Geometry: final body of the model. Coordinates: model frame, mm. Face numbers are marked on the shaded views. A direction names the side the tool comes from. Coordinates: 2 decimals unless noted, no trailing zeros. Order: outer loops, then holes, each group sorted by start corner. A loop starts at its lowest first (then second) coordinate and runs counter-clockwise, first axis right, second up. Notation, with made-up numbers: (-36, -31.5) - (10, -31.5) arc R14 ccw to (10, -5.5) - close; hole circle Ø3 at (84, -4.5). An arc over 180 degrees is marked (long way). Use a Markdown table: item, result. Add a question column.
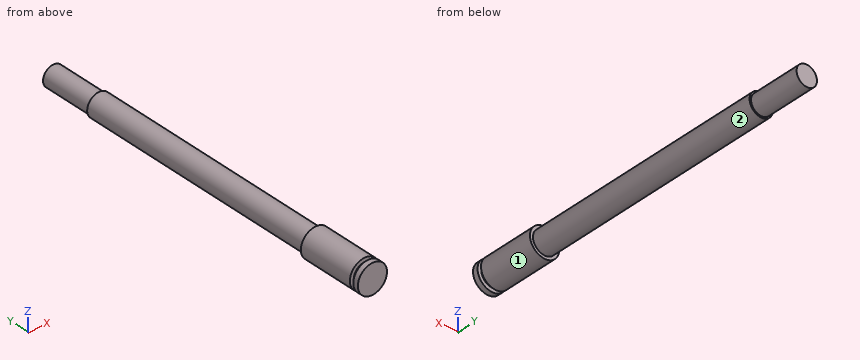
```python
from build123d import *

# Parameters (mm, degrees)
SKETCH1_R           = 5.65
BOSS_EXTRUDE1_DEPTH = 2
SKETCH2_R           = 4.15
BOSS_EXTRUDE2_DEPTH = 1.5
SKETCH3_R           = 5.65
BOSS_EXTRUDE3_DEPTH = 21.5
SKETCH4_R           = 4.5
BOSS_EXTRUDE4_DEPTH = 30
SKETCH5_R           = 4.5
BOSS_EXTRUDE5_DEPTH = 65
SKETCH6_R           = 3.95
BOSS_EXTRUDE6_DEPTH = 20


with BuildPart() as part:
    # Sketch1 → Boss-Extrude1 (new body)
    with BuildSketch(Plane(origin=(0, 0, 0), x_dir=(1, 0, 0), z_dir=(0, 1, 0))):
        with Locations(Location((0, 0, 0), (0, 0, 270))):
            Circle(SKETCH1_R)
    extrude(amount=BOSS_EXTRUDE1_DEPTH)

    # Sketch2 → Boss-Extrude2 (add)
    with BuildSketch(Plane(origin=(0, 2, 0), x_dir=(1, 0, 0), z_dir=(0, 1, 0))):
        with Locations(Location((0, 0, 0), (0, 0, 270))):
            Circle(SKETCH2_R)
    extrude(amount=BOSS_EXTRUDE2_DEPTH)

    # Sketch3 → Boss-Extrude3 (add)
    with BuildSketch(Plane(origin=(0, 3.5, 0), x_dir=(1, 0, 0), z_dir=(0, 1, 0))):
        with Locations(Location((0, 0, 0), (0, 0, 270))):
            Circle(SKETCH3_R)
    extrude(amount=BOSS_EXTRUDE3_DEPTH)

    # Sketch4 → Boss-Extrude4 (add)
    with BuildSketch(Plane(origin=(0, 25, 0), x_dir=(1, 0, 0), z_dir=(0, 1, 0))):
        with Locations(Location((0, 0, 0), (0, 0, 270))):
            Circle(SKETCH4_R)
    extrude(amount=BOSS_EXTRUDE4_DEPTH)

    # Sketch5 → Boss-Extrude5 (add)
    with BuildSketch(Plane(origin=(0, 55, 0), x_dir=(1, 0, 0), z_dir=(0, 1, 0))):
        with Locations(Location((0, 0, 0), (0, 0, 270))):
            Circle(SKETCH5_R)
    extrude(amount=BOSS_EXTRUDE5_DEPTH)

    # Sketch6 → Boss-Extrude6 (add)
    with BuildSketch(Plane(origin=(0, 120, 0), x_dir=(1, 0, 0), z_dir=(0, 1, 0))):
        with Locations(Location((0, 0, 0), (0, 0, 270))):
            Circle(SKETCH6_R)
    extrude(amount=BOSS_EXTRUDE6_DEPTH)


solid = part.part
```
1) Section A-A (x = 0). Return loops of the section in (y, z), then the cut area to 3 significant figures.
2) Section C-C (y = 99). Return loops of the section in (x, z), then the cut area to 3 significant figures.
3) Section D-D (y = 130.5). Return loops of the section in (x, z).
4) Section B-B (z = 0). Return loops of the section in (x, y).
5) Set-up query: the marked faces 1 and 2. Return all of +Z, -Z, +X, -X, +Y, -Y with unobstructed straight access to the full face (end or side cutting, diameter ignored); none if empty.
6) Ray query, line 1 along Y through (x, z) = (-4, -1.5); line 2 along X through (y, z) = (85, 0.5); line 3 along Y through (x, z) = (-3.5, 3). Return the intervals inside material, ascending.
7) Pin query (flat end, axial travel): pin 1 (4 mm diameter, centred on y = 40, z = 4, fed in from +X); pin 2 (1 mm diameter, centred on y = 45, z = -1.5, fed in from +X); pin 3 (2 mm diameter, centred on y = 46.5, z = -1, fed in from -X). Return the tip coordinate at first contact, or that it passes through.
Values follow:
| question | item | result |
|---|---|---|
| 1 | outline | (0, -5.65) - (2, -5.65) - (2, -4.15) - (3.5, -4.15) - (3.5, -5.65) - (25, -5.65) - (25, -4.5) - (120, -4.5) - (120, -3.95) - (140, -3.95) - (140, 3.95) - (120, 3.95) - (120, 4.5) - (25, 4.5) - (25, 5.65) - (3.5, 5.65) - (3.5, 4.15) - (2, 4.15) - (2, 5.65) - (0, 5.65) - close |
| 1 | area | 1,290 mm² |
| 2 | outline | circle Ø9 at (0, 0) |
| 2 | area | 63.6 mm² |
| 3 | outline | circle Ø7.9 at (0, 0) |
| 4 | outline | (-5.65, 0) - (5.65, 0) - (5.65, 2) - (4.15, 2) - (4.15, 3.5) - (5.65, 3.5) - (5.65, 25) - (4.5, 25) - (4.5, 120) - (3.95, 120) - (3.95, 140) - (-3.95, 140) - (-3.95, 120) - (-4.5, 120) - (-4.5, 25) - (-5.65, 25) - (-5.65, 3.5) - (-4.15, 3.5) - (-4.15, 2) - (-5.65, 2) - close |
| 5 | face 1 | +Y, -Y |
| 5 | face 2 | +Y |
| 6 | line 1 | y = 0 to 2, 3.5 to 120 |
| 6 | line 2 | x = -4.47 to 4.47 |
| 6 | line 3 | y = 0 to 2, 3.5 to 25 |
| 7 | pin 1 | stops at x = 4.03 |
| 7 | pin 2 | stops at x = 4.39 |
| 7 | pin 3 | stops at x = -4.5 |
